Geometry check sheet. Reference: drawing and pictorial views, mm from the part's lowest x, y, z. Give positions to 0.01 mm unless a question says otherwise; leave off trailing zeros. Write each loop counter-clockwise with the first axis right and the second up, starting at its lowest first coordinate (ties: lowest second). Pieces come first, ordered by that corner, then holes. Notation, with made-up numbers: M -37,81.5 L 20,81.5 A13 ccw 20,91.5 Z; hole C -16,22 d9. An arc over 180 degrees is marked long. Answer as a JSON object with one key per item and string values.
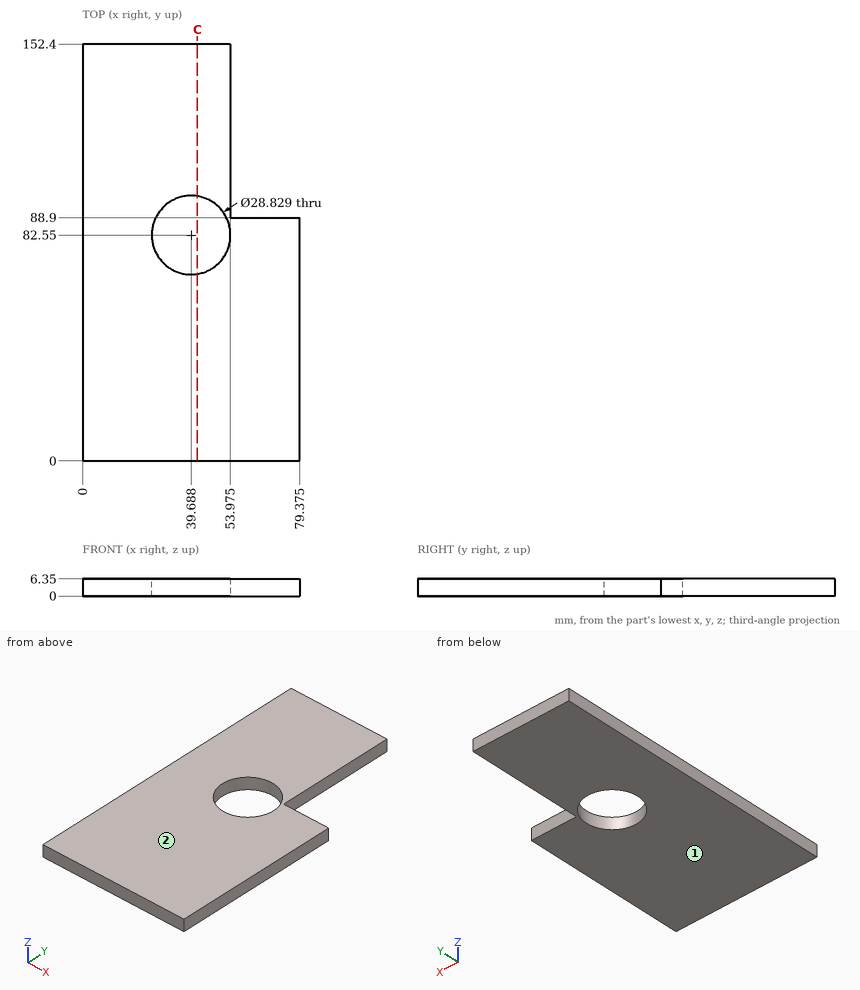
1) Section check C-C on x = 42. Record the boundary of the cut face in (y, z), and give its area (3 significant figures).
Completed:
{"outline": "M 0,0 L 68.32,0 L 68.32,6.35 L 0,6.35 Z; M 96.78,0 L 152.4,0 L 152.4,6.35 L 96.78,6.35 Z", "area": "787 mm2"}
2) Release check for a two-part mould opening along Z. For the marked faces 1 and 2 record: pulls with the +Z half, pulls with the -Z half, needs draft (parallel to the pull), parting line crosses it, or undercut.
Completed:
{"face 1": "pulls with the -Z half", "face 2": "pulls with the +Z half"}
3) Go/stop test with flat-tipped pins: pin 1 (3 mm diameter, centred on x = 33.5, z = 4.5, fed in from -Y); pin 2 (3 mm diameter, centred on x = 62, z = 3, fed in from +Y); pin 3 (1.9 mm diameter, centred on y = 130.5, z = 4, fed in from +X) (1 decimal). Record where each tip stops, or that it passes through.
Completed:
{"pin 1": "stops at y = 0", "pin 2": "stops at y = 88.9", "pin 3": "stops at x = 54"}
4) Thickness scan on L1, parallel to Y at x = 67.5, z = 2.5; L2, parallel to Y at x = 33.5, z = 2.25; L3, parallel to X at y = 84, z = 4.75 (1 decimal). Record the ranges inside material, lowest first.
Completed:
{"L1": "y = 0 to 88.9", "L2": "y = 0 to 69.53, 95.57 to 152.4", "L3": "x = 0 to 25.3, 54 to 79.4"}
